from build123d import *

# Parameters (mm, degrees)
SKETCH1_R                      = 78
BOSS_EXTRUDE1_DEPTH            = 10
BOSS_EXTRUDE2_DEPTH            = 10
FILLET1_R                      = 10
M5_CLEARANCE_HOLE1_D           = 5.5
M5_CLEARANCE_HOLE1_CSINK_D     = 5.55
M5_CLEARANCE_HOLE1_CSINK_ANGLE = 90
CIRPATTERN1_COUNT              = 3
FILLET1_OF_CIRPATTERN1_R       = 10
HOLE1_D                        = 20
HOLE1_CBORE_D                  = 40
HOLE1_CBORE_DEPTH              = 5


with BuildPart() as part:
    # Sketch1 → Boss-Extrude1 (new body)
    with BuildSketch(Plane(origin=(0, 0, 0), x_dir=(1, 0, 0), z_dir=(0, 1, 0))):
        with Locations(Location((0, 0, 0), (0, 0, 270))):
            Circle(SKETCH1_R)
    extrude(amount=BOSS_EXTRUDE1_DEPTH)

    # Sketch4 → Boss-Extrude2 (add)
    with BuildSketch(Plane.XZ):
        with BuildLine():
            Line((-40, 66.962676171), (-40, 266.962676171))
            Line((-40, 266.962676171), (40, 266.962676171))
            Line((40, 266.962676171), (40, 66.962676171))
            ThreePointArc((40, 66.962676171), (0, 78), (-40, 66.962676171))
        make_face()
    boss_extrude2 = extrude(amount=-BOSS_EXTRUDE2_DEPTH)

    # Fillet1
    fillet1_edges = [part.edges().sort_by_distance(p)[0] for p in [
        (40, 5, 266.962676171),
        (-40, 5, 266.962676171),
        (-40, 5, 66.962676171),
        (40, 5, 66.962676171),
    ]]
    fillet(fillet1_edges, radius=FILLET1_R)

    # M5 Clearance Hole1 (through all)
    with Locations(Plane(origin=(0, 10, 0), x_dir=(1, 0, 0), z_dir=(0, 1, 0))):
        with Locations((0, -259.462676171), (-22.5, -236.962676171), (22.5, -236.962676171), (0, -214.462676171)):
            m5_clearance_hole1 = CounterSinkHole(M5_CLEARANCE_HOLE1_D / 2, M5_CLEARANCE_HOLE1_CSINK_D / 2, counter_sink_angle=M5_CLEARANCE_HOLE1_CSINK_ANGLE)

    # CirPattern1: Boss-Extrude2, M5 Clearance Hole1 ×3 about axis
    cirpattern1_axis = Axis((0, 0, 0), (0, 1, 0))
    add([boss_extrude2.rotate(cirpattern1_axis, i * 360 / CIRPATTERN1_COUNT) for i in range(1, CIRPATTERN1_COUNT)])
    add([m5_clearance_hole1.rotate(cirpattern1_axis, i * 360 / CIRPATTERN1_COUNT) for i in range(1, CIRPATTERN1_COUNT)], mode=Mode.SUBTRACT)

    # Fillet1 of CirPattern1
    fillet1_of_cirpattern1_edges = [part.edges().sort_by_distance(p)[0] for p in [
        (211.196459426, 5, -168.122354237),
        (251.196459426, 5, -98.840321934),
        (77.99137867, 5, 1.159678066),
        (37.99137867, 5, -68.122354237),
        (-251.196459426, 5, -98.840321934),
        (-211.196459426, 5, -168.122354237),
        (-37.99137867, 5, -68.122354237),
        (-77.99137867, 5, 1.159678066),
    ]]
    fillet(fillet1_of_cirpattern1_edges, radius=FILLET1_OF_CIRPATTERN1_R)

    # Hole1 (through all)
    with Locations(Plane(origin=(0, 10, 0), x_dir=(1, 0, 0), z_dir=(0, 1, 0))):
        with Locations((0, 0)):
            CounterBoreHole(HOLE1_D / 2, HOLE1_CBORE_D / 2, HOLE1_CBORE_DEPTH)


solid = part.part
Check sheet for the modelled part. Datum: model origin and axes. Units: mm. A direction names the side the tool comes from. Coordinates: 2 decimals unless noted, no trailing zeros. Loops run counter-clockwise (first coordinate to the right, second up) from the corner with the lowest first, then second, coordinate; pieces in that order, holes last. Notation, with made-up numbers: (49.25, 51.5) -> (80.25, 51.5) arc R36 ccw to (80.25, 86.5) -> close; hole circle Ø9 at (84, 21). An arc over 180 degrees is marked (long way). Write item = value, one per line. Start each with the question number.
1. Section check C-C on x = 165. Record the cut outline in (y, z).
2. Tool access check on faces 4 (the flat face through (1, 0, 20)), 5 (the flat face through (-40, 5, 163)), 6 (the flat face through (-121.51, 4.93, -116.34)). Record the directions out of +Z, -Z, +X, -X, +Y, -Y that give a thin tool (end or side, any length) a straight path to the whole face; none if there is none.
3. Draft check along X on faces 1 (the flat face through (0, 5, 266.963)), 2 (the cylindrical face through (0, 5, -78)), 3 (the flat face through (231.406, 4.93, -133.118)). Enter one of: released by +X, released by -X, zero draft, split by the parting line, or undercut.
4. Section check A-A on z = 126. Record the cut outline in (x, y).
5. Depth check by flat-ended pin: P1, Ø1.5, axis at y = 4.5, z = -12, coming from the -X side; P2, Ø5, axis at x = 96, y = 2.5, coming from the +Z side; P3, Ø3.5, axis at x = -224.7, z = -129.73, coming from the -Y side; P4, Ø1, axis at x = 53, y = 3.5, coming from the +Z side. Enter the tip coordinate at first touch or a pass-through.
6. Section check B-B on y = 7.75. Give the number of separate pieces and of enclosed holes in the cut face, then the cut area to 3 significant figures.
7. Material ranges on line 1 (X direction, y = 2.25, z = 233.5); line 2 (Z direction, x = 22.5, y = 3); line 3 (X direction, y = 3.25, z = -138), recorded low to high.
Responses:
q1.outline = (0, -141.45) -> (10, -141.45) -> (10, -49.07) -> (0, -49.07) -> close
q2.face_4 = +Z, -Z, +X, -X, -Y
q2.face_5 = +Z, -X, +Y, -Y
q2.face_6 = -Z, +Y, -Y
q3.face_1 = zero draft
q3.face_2 = undercut
q3.face_3 = released by +X
q4.outline = (-40, 0) -> (40, 0) -> (40, 10) -> (-40, 10) -> close
q5.P1 = -102.08
q5.P2 = -7.79
q5.P3 = through
q5.P4 = 57.69
q6.separate_pieces = 1
q6.enclosed_holes = 13
q6.area = 63,700 mm2
q7.line_1 = -40 to 40
q7.line_2 = -74.68 to 234.21, 239.71 to 266.96
q7.line_3 = -228.59 to -196.72, -191.22 to -159.02, 159.02 to 191.22, 196.72 to 228.59
